The listing builds one solid part. Answer for the finished solid, in the listing's coordinates (mm). Coordinates: 2 decimals unless noted, no trailing zeros. Order: outer loops, then holes, each group sorted by start corner. A loop starts at its lowest first (then second) coordinate and runs counter-clockwise, first axis right, second up. Notation, with made-up numbers: (44, -29) -> (61, -29) arc R12 ccw to (61, -24) -> close; hole circle Ø10 at (-23, 12.25). An arc over 180 degrees is marked (long way). Return JSON: item names as keys, results as strings.
from build123d import *

# Parameters (mm, degrees)
F0_R     = 3.625
F0_R_2   = 11.1
F1_DEPTH = 6.5


with BuildPart() as f1:
    # F0 (on Top) → F1 (new body)
    with BuildSketch(Plane.XY):
        with BuildLine():
            ThreePointArc((-2.8955630067, 13.1858149113), (0, 13.5), (2.8955630067, 13.1858149113))
            ThreePointArc((2.8955630067, 13.1858149113), (4.4428490315, 14.9683455961), (5, 17.2620527446))
            ThreePointArc((5, 17.2620527446), (-2.2937071485, 21.7049017761), (-2.8955630067, 13.1858149113))
        make_face()
        with Locations((0, 17.2620527446)):
            Circle(F0_R, mode=Mode.SUBTRACT)
        with BuildLine():
            ThreePointArc((19.9493761983, -8.6310263723), (17.6501427505, -4.4231931971), (12.8670321861, -4.0852763336))
            ThreePointArc((12.8670321861, -4.0852763336), (11.6913429511, -6.75), (9.9714691794, -9.1005385777))
            ThreePointArc((9.9714691794, -9.1005385777), (15.1843920546, -13.625500073), (19.9493761983, -8.6310263723))
        make_face()
        with Locations((14.9493761983, -8.6310263723)):
            Circle(F0_R, mode=Mode.SUBTRACT)
        with BuildLine():
            ThreePointArc((12.8670321861, -4.0852763336), (13.3408195871, -2.0670105814), (13.5, 0))
            ThreePointArc((13.5, 0), (10.519983379, 8.460493467), (2.8955630067, 13.1858149113))
            ThreePointArc((2.8955630067, 13.1858149113), (0, 12.2620527446), (-2.8955630067, 13.1858149113))
            ThreePointArc((-2.8955630067, 13.1858149113), (-11.6913429511, 6.75), (-12.8670321861, -4.0852763336))
            ThreePointArc((-12.8670321861, -4.0852763336), (-10.7415430231, -5.9302598201), (-9.9493761983, -8.6310263723))
            ThreePointArc((-9.9493761983, -8.6310263723), (-9.9549024976, -8.8660422286), (-9.9714691794, -9.1005385777))
            ThreePointArc((-9.9714691794, -9.1005385777), (0, -13.5), (9.9714691794, -9.1005385777))
            ThreePointArc((9.9714691794, -9.1005385777), (10.6192491794, -6.1310263723), (12.8670321861, -4.0852763336))
        make_face()
        Circle(F0_R_2, mode=Mode.SUBTRACT)
        with BuildLine():
            ThreePointArc((-9.9714691794, -9.1005385777), (-11.6913429511, -6.75), (-12.8670321861, -4.0852763336))
            ThreePointArc((-12.8670321861, -4.0852763336), (-19.2795032172, -11.1310263723), (-9.9714691794, -9.1005385777))
        make_face()
        with Locations((-14.9493761983, -8.6310263723)):
            Circle(F0_R, mode=Mode.SUBTRACT)
        with BuildLine():
            ThreePointArc((9.9714691794, -9.1005385777), (11.6913429511, -6.75), (12.8670321861, -4.0852763336))
            ThreePointArc((12.8670321861, -4.0852763336), (10.6192491794, -6.1310263723), (9.9714691794, -9.1005385777))
        make_face()
        with BuildLine():
            ThreePointArc((-2.8955630067, 13.1858149113), (0, 12.2620527446), (2.8955630067, 13.1858149113))
            ThreePointArc((2.8955630067, 13.1858149113), (0, 13.5), (-2.8955630067, 13.1858149113))
        make_face()
        with BuildLine():
            ThreePointArc((-9.9493761983, -8.6310263723), (-10.7415430231, -5.9302598201), (-12.8670321861, -4.0852763336))
            ThreePointArc((-12.8670321861, -4.0852763336), (-11.6913429511, -6.75), (-9.9714691794, -9.1005385777))
            ThreePointArc((-9.9714691794, -9.1005385777), (-9.9549024976, -8.8660422286), (-9.9493761983, -8.6310263723))
        make_face()
    extrude(amount=F1_DEPTH)


solid = f1.part
1. Each of these flat-tipped pins is pushed along its axis until it touches: pin 1 Ø3 at (y, z) = (-6, 1) entering from +X; pin 2 Ø8 at (x, y) = (14, -2.5) entering from +Z; pin 3 Ø6 at (x, y) = (-14.95, -8.63) entering from +Z; pin 4 Ø1.5 at (y, z) = (-4, 3) entering from +X. Where does it stop, or does it pass through?
Answer block:
{"pin 1": "stops at x = 19.82", "pin 2": "stops at z = 6.5", "pin 3": "passes through", "pin 4": "stops at x = 18.1"}
2. Determine the mould class of faces 1 (the face through (-18.57, -8.47, 3.2)), 2 (the face through (-7.5, 8.4, 0)) for opening direction Y: pulls with the +Y half, pulls with the -Y half, needs draft (parallel to the pull), parting line crosses it, or undercut.
Answer block:
{"face 1": "undercut", "face 2": "needs draft"}
3. The part is cut by section B-B on x = 16.5. Give the vertices of the cut face in (y, z), and give its area (3 significant figures).
Answer block:
{"outline": "(-13.38, 0) -> (-11.91, 0) -> (-11.91, 6.5) -> (-13.38, 6.5) -> close; (-5.35, 0) -> (-3.88, 0) -> (-3.88, 6.5) -> (-5.35, 6.5) -> close", "area": "19.2 mm2"}
4. Consider line 1 (Y direction, x = 0, z = 2); line 2 (Y direction, x = -15, z = 3.5); line 3 (X direction, y = -5.5, z = 4.25). Determine where each line is inside the solid, lowest interval first. Write a range as from..to.
Answer block:
{"line 1": "y = -13.5..-11.1, 11.1..13.64, 20.89..22.26", "line 2": "y = -13.63..-12.26, -5.01..-3.63", "line 3": "x = -18.85..-16.78, -13.12..-9.64, 9.64..13.12, 16.78..18.85"}
5. The part is cut by section D-D on y = -7. Give the vertices of the cut face in (x, z), and give its area (3 significant figures).
Answer block:
{"outline": "(-19.68, 0) -> (-18.19, 0) -> (-18.19, 6.5) -> (-19.68, 6.5) -> close; (-11.71, 0) -> (-8.61, 0) -> (-8.61, 6.5) -> (-11.71, 6.5) -> close; (8.61, 0) -> (11.71, 0) -> (11.71, 6.5) -> (8.61, 6.5) -> close; (18.19, 0) -> (19.68, 0) -> (19.68, 6.5) -> (18.19, 6.5) -> close", "area": "59.6 mm2"}
6. The part is cut by section A-A on x = 0. Give the vertices of the cut face in (y, z).
Answer block:
{"outline": "(-13.5, 0) -> (-11.1, 0) -> (-11.1, 6.5) -> (-13.5, 6.5) -> close; (11.1, 0) -> (13.64, 0) -> (13.64, 6.5) -> (11.1, 6.5) -> close; (20.89, 0) -> (22.26, 0) -> (22.26, 6.5) -> (20.89, 6.5) -> close"}
7. The part is cut by section C-C on z = 3.5. Give the vertices of the cut face in (x, y) (3 decimals), and give its area (3 significant figures).
Answer block:
{"outline": "(-12.867, -4.085) arc R5 ccw (long way) to (-9.971, -9.101) arc R13.5 ccw to (9.971, -9.101) arc R5 ccw (long way) to (12.867, -4.085) arc R13.5 ccw to (2.896, 13.186) arc R5 ccw (long way) to (-2.896, 13.186) arc R13.5 ccw to start; hole circle Ø7.25 at (-14.949, -8.631); hole circle Ø22.2 at (0, 0); hole circle Ø7.25 at (0, 17.262); hole circle Ø7.25 at (14.949, -8.631)", "area": "283 mm2"}
